Input: part model. Units: mm. Frame: model coordinates. A direction names the side the tool comes from. Round coordinates to 2 decimals unless told otherwise and drop trailing zeros. Loops run counter-clockwise (first coordinate to the right, second up) from the corner with the lowest first, then second, coordinate; pieces in that order, holes last.
(1) Line query: line 1 (Y direction, x = 0, z = 3); line 2 (Z direction, x = 9.5, y = -10.5); line 3 (Z direction, x = 7, y = 6). Output: solid intervals per line, ascending.
(2) Draft query along X for faces 4 (the face through (2.38, -10.74, -0.99)), 5 (the face through (0, -14, 5)), 6 (the face through (-8, -8, 0)). Return one class per face: released by +X, released by -X, zero draft, split by the parting line, or undercut.
(3) Cut plane A-A, the plane x = 0. Output: boundary loops of the cut face in (y, z).
(4) Cut plane B-B, the plane y = 14. Output: boundary loops of the cut face in (x, z).
(5) First-contact query: pin 1 Ø1.8 at (x, y) = (-14, 0) entering from -Z; pin 2 Ø1.5 at (y, z) = (14, 36.5) entering from +X; pin 3 Ø1.5 at (y, z) = (12.5, 2.5) entering from -X; pin 4 Ø12 at (y, z) = (13.5, -7.5) entering from +X. Flat tips, straight axial feed; report the tip coordinate or a pass-through.
(6) Access query for faces 1 (the face through (-3.772, -16.986, 47.283)), 2 (the face through (0, 0, 63)), 3 (the face through (-12.5, 0.07, 2.46)). Directions: +Z, -Z, +X, -X, +Y, -Y. A direction counts if a zero-diameter tool reaches every point of the face in a straight line with its end or side. Return the directions, or none.
(7) Cut plane C-C, the plane z = 31. Output: boundary loops of the cut face in (x, y), and give its area (3 significant figures).
from build123d import *

# Parameters (mm, degrees)
SKETCH_1_R          = 18
EXTRUDE_1_DEPTH     = 32
SKETCH_2_R          = 17.4
EXTRUDE_2_DEPTH     = 31
SKETCH_3_R          = 11
EXTRUDE_3_DEPTH     = 2
SKETCH_4_R          = 4
EXTRUDE_4_DEPTH     = 3
SKETCH_5_R          = 3
EXTRUDE_5_DEPTH     = 15
SKETCH_6_R          = 1.5
CUT_EXTRUDE_2_DEPTH = 5


with BuildPart() as part:
    # 草图1 → 凸台-拉伸1 (new body)
    with BuildSketch(Plane.XY):
        Circle(SKETCH_1_R)
    extrude(amount=EXTRUDE_1_DEPTH)

    # 草图2 → 凸台-拉伸2 (add)
    with BuildSketch(Plane.XY.offset(32)):
        Circle(SKETCH_2_R)
    extrude(amount=EXTRUDE_2_DEPTH)

    # 草图3 → 凸台-拉伸3 (add)
    with BuildSketch(Plane(origin=(0, 0, 0), x_dir=(-1, 0, 0), z_dir=(0, 0, -1))):
        Circle(SKETCH_3_R)
    extrude(amount=EXTRUDE_3_DEPTH)

    # 草图4 → 凸台-拉伸4 (add)
    with BuildSketch(Plane(origin=(0, 0, -2), x_dir=(-1, 0, 0), z_dir=(0, 0, -1))):
        Circle(SKETCH_4_R)
    extrude(amount=EXTRUDE_4_DEPTH)

    # 草图5 → 凸台-拉伸5 (add)
    with BuildSketch(Plane(origin=(0, 0, -5), x_dir=(-1, 0, 0), z_dir=(0, 0, -1))):
        Circle(SKETCH_5_R)
    extrude(amount=EXTRUDE_5_DEPTH)

    # 草图6 → 切除-拉伸2 (cut)
    with BuildSketch(Plane(origin=(0, 0, 0), x_dir=(-1, 0, 0), z_dir=(0, 0, -1))):
        with Locations((0, 14)):
            Circle(SKETCH_6_R)
        with Locations((0, -14)):
            Circle(SKETCH_6_R)
        with Locations((14, 0)):
            Circle(SKETCH_6_R)
        with Locations((-14, 0)):
            Circle(SKETCH_6_R)
    extrude(amount=-CUT_EXTRUDE_2_DEPTH, mode=Mode.SUBTRACT)


solid = part.part
Reported:
1. line 1: y = -18 to -15.5, -12.5 to 12.5, 15.5 to 18
1. line 2: z = 0 to 63
1. line 3: z = -2 to 63
2. face 4: split by the parting line
2. face 5: undercut
2. face 6: zero draft
3. outline: (-18, 0) - (-15.5, 0) - (-15.5, 5) - (-12.5, 5) - (-12.5, 0) - (-11, 0) - (-11, -2) - (-4, -2) - (-4, -5) - (-3, -5) - (-3, -20) - (3, -20) - (3, -5) - (4, -5) - (4, -2) - (11, -2) - (11, 0) - (12.5, 0) - (12.5, 5) - (15.5, 5) - (15.5, 0) - (18, 0) - (18, 32) - (17.4, 32) - (17.4, 63) - (-17.4, 63) - (-17.4, 32) - (-18, 32) - close
4. outline: (-11.31, 0) - (-1.5, 0) - (-1.5, 5) - (1.5, 5) - (1.5, 0) - (11.31, 0) - (11.31, 32) - (10.33, 32) - (10.33, 63) - (-10.33, 63) - (-10.33, 32) - (-11.31, 32) - close
5. pin 1: stops at z = 5
5. pin 2: stops at x = 11.28
5. pin 3: stops at x = -13.64
5. pin 4: passes through
6. face 1: +Z
6. face 2: +Z, +X, -X, +Y, -Y
6. face 3: -Z
7. outline: circle Ø36 at (0, 0)
7. area: 1,020 mm2
